For this review, take the finished solid that the model builds, in its own axes (mm). Give positions to 0.01 mm unless a question says otherwise; leave off trailing zeros.
Q1. For line 1 (X direction, y = 0.6, z = 38) (3 decimals); line 2 (X direction, y = 1.6, z = -37.5), list the stretches that pass through material, from the lowest coordinate up.
Q2. Insertion check: P1, Ø2.5, axis at x = -63, z = 38, coming from the -Y side. The pin has a flat end and moves straight along its axis. Give the tip position at first contact, or say it passes through.
Q3. Mouldability with a two-part tool opening along X and no side actions: class faces 1 (the flat face through (-1, 1, -50)), 2 (the flat face through (75, 1, 1)), 3 (the cylindrical face through (-61.8, 1.52, -37.23)) as released by +X, released by -X, zero draft, split by the parting line, or undercut.
```python
from build123d import *

# Parameters (mm, degrees)
SKETCH1_W           = 150
SKETCH1_H           = 100
BOSS_EXTRUDE1_DEPTH = 3
SKETCH2_R           = 1.425
CUT_EXTRUDE1_DEPTH  = 10
LPATTERN1_COUNT     = 2
LPATTERN1_PITCH     = 76


with BuildPart() as part:
    # Sketch1 → Boss-Extrude1 (new body)
    with BuildSketch(Plane(origin=(0, 0, 0), x_dir=(1, 0, 0), z_dir=(0, 1, 0))):
        Rectangle(SKETCH1_W, SKETCH1_H)
    extrude(amount=BOSS_EXTRUDE1_DEPTH)

    # Sketch2 → Cut-Extrude1 (cut)
    with BuildSketch(Plane(origin=(0, 3, 0), x_dir=(1, 0, 0), z_dir=(0, 1, 0))):
        with Locations(Location((-63, 38, 0), (0, 0, 270))):
            Circle(SKETCH2_R)
    cut_extrude1 = extrude(amount=-CUT_EXTRUDE1_DEPTH, mode=Mode.SUBTRACT)

    # LPattern1: Cut-Extrude1 ×2
    with Locations(*[(0, 0, i * LPATTERN1_PITCH) for i in range(1, LPATTERN1_COUNT)]):
        add(cut_extrude1, mode=Mode.SUBTRACT)


solid = part.part
```
Computed:
1. line 1: x = -75 to -64.425, -61.575 to 75
1. line 2: x = -75 to -64.33, -61.67 to 75
2. P1: passes through
3. face 1: zero draft
3. face 2: released by +X
3. face 3: undercut
